Read the model definition and answer for the solid it produces. Units are mm, in the model's axes. A direction names the side the tool comes from. Give positions to 0.01 mm unless a question says otherwise; leave off trailing zeros. Order: outer loops, then holes, each group sorted by start corner. A loop starts at its lowest first (then second) coordinate and runs counter-clockwise, first axis right, second up.
Item 1: A cutting plane is placed at D-D (x = 10). Write down the section's boundary in (y, z), plus the area to 3 significant figures.
Item 2: A cutting plane is placed at A-A (y = -8). Write down the section's boundary in (x, z).
Item 3: Given pin 1 Ø2 at (x, y) = (-12.5, -2.5) entering from -Z; pin 2 Ø1 at (x, y) = (-2, 2.5) entering from +Z, each flat-ended and moving along its own axis, determine where each tip first touches the part or whether it passes through.
Item 4: Which of the six approach directions +Z, -Z, +X, -X, +Y, -Y give full straight-line access (tool end or side, diameter ignored) to faces 4 (the face through (6.386, -0.575, 42.986)), 5 (the face through (12.5, -0.1, 39)), 6 (the face through (10, 0, 44))?
Item 5: The mould has two halves that part along Y. Classify faces 1 (the face through (0, 0, 36)), 2 (the face through (0, 0, 43)), 3 (the face through (13.5, 0.07, 42.99)): +Y half, -Y half, draft (parallel to the pull), parting line (faces both ways), or undercut.
Item 6: Find the intervals of material crossed by line 1 along Z through (x, y) = (5, 8.5); line 2 along Z through (x, y) = (5, -8.75); line 3 along Y through (x, z) = (5, 43), in increasing order.
Item 7: A cutting plane is placed at B-B (y = 0). Write down the section's boundary in (x, z), plus the area to 3 significant figures.
Item 8: A cutting plane is placed at C-C (x = 15). Write down the section's boundary in (y, z), plus the area to 3 significant figures.
from build123d import *

# Parameters (mm, degrees)
SKETCH_1_W      = 40
SKETCH_1_H      = 20
EXTRUDE_1_DEPTH = 36
SKETCH_2_R      = 2.5
EXTRUDE_2_DEPTH = 6
SKETCH_4_R      = 10
SKETCH_4_R_2    = 1.5
EXTRUDE_3_DEPTH = 2


with BuildPart() as part:
    # Эскиз1 → Бобышка-Вытянуть1 (new body)
    with BuildSketch(Plane.XY):
        Rectangle(SKETCH_1_W, SKETCH_1_H)
    extrude(amount=EXTRUDE_1_DEPTH)

    # Эскиз2 → Бобышка-Вытянуть2 (add)
    with BuildSketch(Plane.XY.offset(36)):
        with Locations(Location((10, 0, 0), (0, 0, 180))):
            Circle(SKETCH_2_R)
    extrude(amount=EXTRUDE_2_DEPTH)

    # Эскиз4 → Бобышка-Вытянуть3 (add)
    with BuildSketch(Plane.XY.offset(42)):
        with Locations((10, 0)):
            Circle(SKETCH_4_R)
        with Locations((5, 0)):
            Circle(SKETCH_4_R_2, mode=Mode.SUBTRACT)
        with Locations((15, 0)):
            Circle(SKETCH_4_R_2, mode=Mode.SUBTRACT)
    extrude(amount=EXTRUDE_3_DEPTH)


solid = part.part
Response values:
1. outline: (-10, 0) - (10, 0) - (10, 36) - (2.5, 36) - (2.5, 42) - (10, 42) - (10, 44) - (-10, 44) - (-10, 42) - (-2.5, 42) - (-2.5, 36) - (-10, 36) - close
1. area: 790 mm2
2. outline: (-20, 0) - (20, 0) - (20, 36) - (-20, 36) - close; (4, 42) - (16, 42) - (16, 44) - (4, 44) - close
3. pin 1: stops at z = 0
3. pin 2: stops at z = 36
4. face 4: +Z
4. face 5: none
4. face 6: +Z, +X, -X, +Y, -Y
5. face 1: draft
5. face 2: parting line
5. face 3: undercut
6. line 1: z = 0 to 36, 42 to 44
6. line 2: z = 0 to 36
6. line 3: y = -8.66 to -1.5, 1.5 to 8.66
7. outline: (-20, 0) - (20, 0) - (20, 36) - (12.5, 36) - (12.5, 42) - (13.5, 42) - (13.5, 44) - (6.5, 44) - (6.5, 42) - (7.5, 42) - (7.5, 36) - (-20, 36) - close; (0, 42) - (3.5, 42) - (3.5, 44) - (0, 44) - close; (16.5, 42) - (20, 42) - (20, 44) - (16.5, 44) - close
7. area: 1,500 mm2
8. outline: (-10, 0) - (10, 0) - (10, 36) - (-10, 36) - close; (-8.66, 42) - (-1.5, 42) - (-1.5, 44) - (-8.66, 44) - close; (1.5, 42) - (8.66, 42) - (8.66, 44) - (1.5, 44) - close
8. area: 749 mm2
